from build123d import *

# Parameters (mm, degrees)
SKETCH1_W           = 384.683
SKETCH1_H           = 174.244
BOSS_EXTRUDE1_DEPTH = 6.35
CUT_EXTRUDE1_REACH  = 1839.085
SKETCH2_R           = 11.1125
CUT_EXTRUDE2_REACH  = 1839.085
SKETCH3_W           = 7.14375
SKETCH3_H           = 90.297


with BuildPart() as part:
    # Sketch1 → Boss-Extrude1 (new body)
    with BuildSketch(Plane.XY):
        with Locations((1630.751253019, 139.093604852)):
            Rectangle(SKETCH1_W, SKETCH1_H)
    extrude(amount=BOSS_EXTRUDE1_DEPTH)

    # Sketch2 → Cut-Extrude1 (cut, up to next)
    with BuildSketch(Plane.XY.offset(6.35), mode=Mode.PRIVATE) as cut_extrude1_sk1:
        with Locations((1778.642753019, 196.243604852)):
            Circle(SKETCH2_R)
    cut_extrude1_tool1 = extrude(cut_extrude1_sk1.sketch, amount=-CUT_EXTRUDE1_REACH, mode=Mode.PRIVATE) & part.part
    # Sketch2 → Cut-Extrude1 (cut, up to next)
    with BuildSketch(Plane.XY.offset(6.35), mode=Mode.PRIVATE) as cut_extrude1_sk2:
        with Locations((1778.642753019, 81.943604852)):
            Circle(SKETCH2_R)
    cut_extrude1_tool2 = extrude(cut_extrude1_sk2.sketch, amount=-CUT_EXTRUDE1_REACH, mode=Mode.PRIVATE) & part.part
    # Sketch2 → Cut-Extrude1 (cut, up to next)
    with BuildSketch(Plane.XY.offset(6.35), mode=Mode.PRIVATE) as cut_extrude1_sk3:
        with Locations((1482.859753019, 196.243604852)):
            Circle(SKETCH2_R)
    cut_extrude1_tool3 = extrude(cut_extrude1_sk3.sketch, amount=-CUT_EXTRUDE1_REACH, mode=Mode.PRIVATE) & part.part
    # Sketch2 → Cut-Extrude1 (cut, up to next)
    with BuildSketch(Plane.XY.offset(6.35), mode=Mode.PRIVATE) as cut_extrude1_sk4:
        with Locations((1482.859753019, 81.943604852)):
            Circle(SKETCH2_R)
    cut_extrude1_tool4 = extrude(cut_extrude1_sk4.sketch, amount=-CUT_EXTRUDE1_REACH, mode=Mode.PRIVATE) & part.part
    add(cut_extrude1_tool1.solids().sort_by_distance((1778.642753, 196.243605, 6.35))[0], mode=Mode.SUBTRACT)
    add(cut_extrude1_tool2.solids().sort_by_distance((1778.642753, 81.943605, 6.35))[0], mode=Mode.SUBTRACT)
    add(cut_extrude1_tool3.solids().sort_by_distance((1482.859753, 196.243605, 6.35))[0], mode=Mode.SUBTRACT)
    add(cut_extrude1_tool4.solids().sort_by_distance((1482.859753, 81.943605, 6.35))[0], mode=Mode.SUBTRACT)

    # Sketch3 → Cut-Extrude2 (cut, up to next)
    with BuildSketch(Plane.XY.offset(6.35), mode=Mode.PRIVATE) as cut_extrude2_sk1:
        with Locations((1638.371253019, 181.067104852)):
            Rectangle(SKETCH3_W, SKETCH3_H)
    cut_extrude2_tool1 = extrude(cut_extrude2_sk1.sketch, amount=-CUT_EXTRUDE2_REACH, mode=Mode.PRIVATE) & part.part
    add(cut_extrude2_tool1.solids().sort_by_distance((1638.371253, 181.067105, 6.35))[0], mode=Mode.SUBTRACT)


solid = part.part
Model file for the job. Use its own axes, mm. A direction names the side the tool comes from. Round coordinates to 2 decimals unless told otherwise and drop trailing zeros. Loops run counter-clockwise (first coordinate to the right, second up) from the corner with the lowest first, then second, coordinate; pieces in that order, holes last. Notation, with made-up numbers: M -32,65.25 L 15,65.25 A18 cw 15,80.25 Z; hole C 77.25,76.5 d9. An arc over 180 degrees is marked long. One line per question, with ' | ' between items.
1) Flat gauge pin, fed straight in: pin 1 (3 mm diameter, centred on x = 1636.5, z = 4.5, fed in from +Y). Where does the tip first touch, or does it go through?
Solved:
pin 1: stops at y = 135.92
2) Band-saw the part on A-A (y = 180). Give the cut face in (x, z), then the cut area to 3 significant figures.
Solved:
outline: M 1438.41,0 L 1634.8,0 L 1634.8,6.35 L 1438.41,6.35 Z; M 1641.94,0 L 1823.09,0 L 1823.09,6.35 L 1641.94,6.35 Z | area: 2,400 mm²
3) Drill centre lines: line 1 along X through (y, z) = (164.5, 3.75); line 2 along X through (y, z) = (82, 4.25); line 3 along X through (y, z) = (204, 2.5) (3 decimals). Where is each one in solid material? Low to high.
Solved:
line 1: x = 1438.41 to 1634.8, 1641.94 to 1823.09 | line 2: x = 1438.41 to 1471.75, 1493.97 to 1767.53, 1789.76 to 1823.09 | line 3: x = 1438.41 to 1474.902, 1490.818 to 1634.799, 1641.943 to 1770.685, 1786.601 to 1823.093
4) Mould opens along X. For faces 1 (the flat face through (1823.093, 138, 3)), 2 (the flat face through (1638, 135.919, 3)), 3 (the flat face through (1628, 140, 0)) say: +X half, -X half, draft (parallel to the pull), parting line (faces both ways), or undercut.
Solved:
face 1: +X half | face 2: undercut | face 3: draft
5) Band-saw the part on B-B (z = 3). Give the cut face in (x, y) (1 decimal).
Solved:
outline: M 1438.4,52 L 1823.1,52 L 1823.1,226.2 L 1641.9,226.2 L 1641.9,135.9 L 1634.8,135.9 L 1634.8,226.2 L 1438.4,226.2 Z; hole C 1482.9,81.9 d22.2; hole C 1482.9,196.2 d22.2; hole C 1778.6,81.9 d22.2; hole C 1778.6,196.2 d22.2
6) 3-axis set-ups, long thin cutter, end or side, ignore diameter. For faces 4 (the flat face through (1641.943, 180, 3)), 5 (the cylindrical face through (1767.54, 82.43, 3.22)): which of +Z, -Z, +X, -X, +Y, -Y reach the whole face in a straight line?
Solved:
face 4: +Z, -Z, +Y | face 5: +Z, -Z
